Here's how the part is built. I have some questions about the finished solid (model axes, mm). A direction names the side the tool comes from. Round coordinates to 2 decimals unless told otherwise and drop trailing zeros. Write each loop counter-clockwise with the first axis right and the second up, starting at its lowest first coordinate (ties: lowest second). Pieces come first, ordered by that corner, then holes. Notation, with made-up numbers: (-36.75, -2) -> (6.25, -2) arc R10 ccw to (6.25, 2) -> close; hole circle Ø7 at (16, 32.5). An arc over 180 degrees is marked (long way). Answer in a Markdown table with one row per item.
from build123d import *

# Parameters (mm, degrees)
F0_R     = 50.8
F0_W     = 25.4
F0_H     = 127
F1_DEPTH = 25.4
F2_DEPTH = 431.8


with BuildPart() as f1:
    # F0 (on Top) → F1 (new body)
    with BuildSketch(Plane.XY):
        Polygon((-190.5, 508), (-190.5, 381), (-12.7, 381), (12.7, 381), (190.5, 381), (190.5, 508), align=None)
        Polygon((190.5, 381), (12.7, 381), (12.7, 254), (12.7, 127), (12.7, 0), (12.7, -127), (12.7, -254), (12.7, -381), (190.5, -381), align=None)
        Polygon((849.801779, 508), (190.5, 508), (190.5, 381), (190.5, -381), (849.801779, -381), align=None)
        with Locations((520.150889, -228.6)):
            Circle(F0_R, mode=Mode.SUBTRACT)
        with Locations((520.150889, 355.6)):
            Circle(F0_R, mode=Mode.SUBTRACT)
        with Locations((520.150889, 355.6)):
            Circle(F0_R)
        with Locations((520.150889, -228.6)):
            Circle(F0_R)
        Polygon((-12.7, 381), (-190.5, 381), (-190.5, -381), (-12.7, -381), (-12.7, -254), (-12.7, -127), (-12.7, 0), (-12.7, 127), (-12.7, 254), align=None)
        Polygon((-190.5, -381), (-190.5, 381), (-190.5, 508), (-849.801779, 508), (-849.801779, -381), align=None)
        with Locations((-520.150889, -228.6)):
            Circle(F0_R, mode=Mode.SUBTRACT)
        with Locations((-520.150889, 355.6)):
            Circle(F0_R, mode=Mode.SUBTRACT)
        with Locations((-520.150889, 355.6)):
            Circle(F0_R)
        with Locations((-520.150889, -228.6)):
            Circle(F0_R)
        with Locations((0, -317.5)):
            Rectangle(F0_W, F0_H)
        with Locations((0, -190.5)):
            Rectangle(F0_W, F0_H)
        with Locations((0, -63.5)):
            Rectangle(F0_W, F0_H)
        with Locations((0, 63.5)):
            Rectangle(F0_W, F0_H)
        with Locations((0, 317.5)):
            Rectangle(F0_W, F0_H)
        with Locations((0, 190.5)):
            Rectangle(F0_W, F0_H)
    extrude(amount=F1_DEPTH)

    # F0 (on Top) → F2 (join)
    with BuildSketch(Plane.XY):
        with Locations((-520.150889, 355.6)):
            Circle(F0_R)
        with Locations((520.150889, 355.6)):
            Circle(F0_R)
        with Locations((520.150889, -228.6)):
            Circle(F0_R)
        with Locations((-520.150889, -228.6)):
            Circle(F0_R)
    extrude(amount=F2_DEPTH)


solid = f1.part
1) I want a section at A-A, the plane z = 57. List the corners of the cut face in (x, y) for me, and give its area (3 significant figures).
Response:
| item | result |
|---|---|
| outline | circle Ø101.6 at (-520.15, -228.6); circle Ø101.6 at (-520.15, 355.6); circle Ø101.6 at (520.15, -228.6); circle Ø101.6 at (520.15, 355.6) |
| area | 32,400 mm^2 |
2) I want a section at B-B, the plane y = 355.6. List the corners of the cut face in (x, z) for me, and give its area (3 significant figures).
Response:
| item | result |
|---|---|
| outline | (-849.8, 0) -> (849.8, 0) -> (849.8, 25.4) -> (570.95, 25.4) -> (570.95, 431.8) -> (469.35, 431.8) -> (469.35, 25.4) -> (-469.35, 25.4) -> (-469.35, 431.8) -> (-570.95, 431.8) -> (-570.95, 25.4) -> (-849.8, 25.4) -> close |
| area | 126,000 mm^2 |
3) We'd pull the mould along Y, two halves only. Please class faces 3 (the face through (-471.697, -213.341, 225.755)), 4 (the face through (-521, -228, 431.8)): +Y half, -Y half, draft (parallel to the pull), parting line (faces both ways), or undercut.
Response:
| item | result |
|---|---|
| face 3 | undercut |
| face 4 | draft |
4) I want a section at D-D, the plane y = -80. List the corners of the cut face in (x, z) for me, and give its area (3 significant figures).
Response:
| item | result |
|---|---|
| outline | (-849.8, 0) -> (849.8, 0) -> (849.8, 25.4) -> (-849.8, 25.4) -> close |
| area | 43,200 mm^2 |
5) I need wall thicknesses on line 1 (Y direction, x = -518.5, z = 31.5); line 2 (Z direction, x = 352, y = 68.5); line 3 (X direction, y = -189.5, z = 229.5). Which ranges of each line are inside material? Lowest first, please. Write a range as [from, to].
Response:
| item | result |
|---|---|
| line 1 | y = [-279.37, -177.83], [304.83, 406.37] |
| line 2 | z = [0, 25.4] |
| line 3 | x = [-552.58, -487.72], [487.72, 552.58] |
6) Which directions (+Z, -Z, +X, -X, +Y, -Y) give clear straight access to the entire face, cutting with the end or side of a thin tool? Please do faces 1 (the face through (568.605, 370.859, 225.755)), 2 (the face through (-12, 70, 0)).
Response:
| item | result |
|---|---|
| face 1 | +Z |
| face 2 | -Z, +X, -X, +Y, -Y |
7) I want a section at C-C, the plane x = -538. List the corners of the cut face in (y, z) for me, and give its area (3 significant figures).
Response:
| item | result |
|---|---|
| outline | (-381, 0) -> (508, 0) -> (508, 25.4) -> (403.16, 25.4) -> (403.16, 431.8) -> (308.04, 431.8) -> (308.04, 25.4) -> (-181.04, 25.4) -> (-181.04, 431.8) -> (-276.16, 431.8) -> (-276.16, 25.4) -> (-381, 25.4) -> close |
| area | 99,900 mm^2 |
8) For pin 1 (1 mm diameter, centred on x = 263, y = 119, fed in from +Z); pin 2 (2 mm diameter, centred on x = -511.5, z = 111, fed in from -Y); pin 3 (10 mm diameter, centred on y = -212, z = 99.5, fed in from +X), each with a flat end and sliding along its axis, tell me the tip position at first contact or that it passes through.
Response:
| item | result |
|---|---|
| pin 1 | stops at z = 25.4 |
| pin 2 | stops at y = -278.82 |
| pin 3 | stops at x = 569.61 |
